Work out the finished part from the listing and answer in its coordinate system (mm). Face numbers are marked on the shaded views. A direction names the side the tool comes from. Round coordinates to 2 decimals unless told otherwise and drop trailing zeros. Write each loop counter-clockwise with the first axis right and the second up, starting at its lowest first coordinate (ties: lowest second). Pieces come first, ordered by that corner, then holes. Notation, with made-up numbers: (59, 39.5) -> (90, 39.5) arc R16 cw to (90, 52.5) -> close; hole circle Ø10 at (86.5, -39.75). An arc over 180 degrees is marked (long way). One line per item, written item: value.
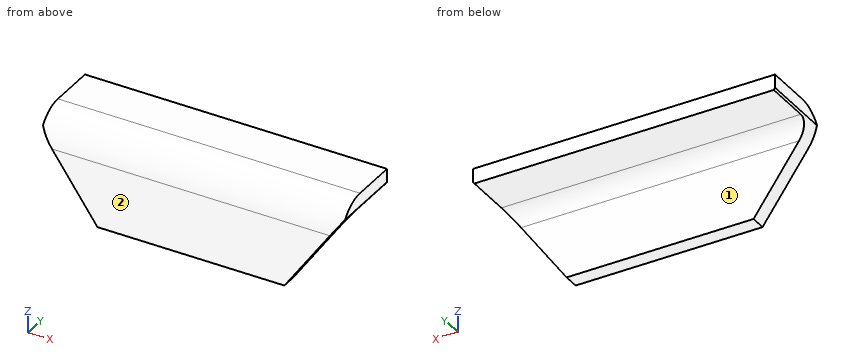
```python
from build123d import *

# Parameters (mm, degrees)
SKETCH1_W                    = 158
SKETCH1_H                    = 50
BASE_FLANGE1_DEPTH           = 8
EDGE_FLANGE1_STRIP_W         = 48
EDGE_FLANGE1_STRIP_H         = 8
EDGE_FLANGE1_STRIP_CUT_DEPTH = 158
EDGE_FLANGE1_DEPTH           = 158
CHAMFER1_SIZE                = 43
CHAMFER1_SIZE2               = 30.108924143
MIRROR2_START                = 54.388635645
MIRROR2_OUTLINE_W            = 56
MIRROR2_OUTLINE_H            = 41
MIRROR2_DEPTH                = 24.663786763


# Read off the part's stored shape, not the designer's step: Mirror2
# Sheet-metal steps are written as plain solids
with BuildPart() as part:
    # Sketch1 → Base-Flange1 (new body)
    with BuildSketch(Plane(origin=(0, 0, 0), x_dir=(1, 0, 0), z_dir=(0, 1, 0))):
        Rectangle(SKETCH1_W, SKETCH1_H)
    extrude(amount=-BASE_FLANGE1_DEPTH)

    # Edge-Flange1 strip (across the edge) → Edge-Flange1 strip cut (cut)
    with BuildSketch(Plane(origin=(-79, 0, 25), x_dir=(0, 0, -1), z_dir=(1, 0, 0))):
        with Locations((-8, -4)):
            Rectangle(EDGE_FLANGE1_STRIP_W, EDGE_FLANGE1_STRIP_H)
    extrude(amount=EDGE_FLANGE1_STRIP_CUT_DEPTH, mode=Mode.SUBTRACT)

    # Edge-Flange1 section (across the edge) → Edge-Flange1 (add)
    with BuildSketch(Plane(origin=(-79, 0, 25), x_dir=(0, 0, -1), z_dir=(1, 0, 0))):
        with BuildLine():
            Line((0, 8), (0, 32))
            Line((0, 32), (8, 32))
            Line((8, 32), (8, 8))
            ThreePointArc((8, 8), (10.343145751, 2.343145751), (16, 0))
            Line((16, 0), (16, -8))
            ThreePointArc((16, -8), (4.686291501, -3.313708499), (0, 8))
        make_face()
    extrude(amount=EDGE_FLANGE1_DEPTH)

    # Chamfer1
    chamfer1_edges = [part.edges().sort_by_distance(p)[0] for p in [
        (-79, -4, -25),
    ]]
    chamfer1_side = [part.faces().sort_by_distance(p)[0] for p in [
        (-79, -0.640312424, -8),
    ]]
    chamfer(chamfer1_edges, length=CHAMFER1_SIZE, length2=CHAMFER1_SIZE2, reference=chamfer1_side[0])

    # Mirror2 outline → Mirror2 (cut)
    with BuildSketch(Plane(origin=(0, 0, 0), x_dir=(0.5735764363510512, 0, 0.8191520442889882), z_dir=(0.8191520442889882, 0, -0.5735764363510512)).offset(MIRROR2_START)):
        with Locations((34, -12.5)):
            Rectangle(MIRROR2_OUTLINE_W, MIRROR2_OUTLINE_H)
    extrude(amount=MIRROR2_DEPTH, mode=Mode.SUBTRACT)


solid = part.part
```
(1) Find section C-C on y = 22.5. Give the vertices of the cut face in (x, z).
Reported:
outline: (-79, 18) -> (-78.3, 17) -> (78.3, 17) -> (79, 18) -> (79, 25) -> (-79, 25) -> close
(2) Find section D-D on z = -17.5. Give the vertices of the cut face in (x, y), plus the area to 3 significant figures.
Reported:
outline: (-54.14, -8) -> (54.14, -8) -> (54.14, 0) -> (-54.14, 0) -> close
area: 866 mm2
(3) Find section A-A on x = 18. Give the vertices of the cut face in (y, z), plus the area to 3 significant figures.
Reported:
outline: (-8, -25) -> (0, -25) -> (0, 9) arc R8 cw to (8, 17) -> (32, 17) -> (32, 25) -> (8, 25) arc R16 ccw to (-8, 9) -> close
area: 615 mm2
(4) Flat-ended cylindrical pins translate along their axes: pin 1 Ø10 at (y, z) = (-0.5, 8) entering from +X; pin 2 Ø8 at (x, z) = (-24.5, 6.5) entering from +Y; pin 3 Ø2 at (y, z) = (-3.5, 16) entering from +X. Find the tip coordinate at first contact, or state that the pin passes through.
Reported:
pin 1: stops at x = 75.5
pin 2: stops at y = 0.14
pin 3: stops at x = 78.3
(5) Find section B-B on y = -2. Give the vertices of the cut face in (x, z), plus the area to 3 significant figures.
Reported:
outline: (-79, 18) -> (-48.89, -25) -> (48.89, -25) -> (79, 18) -> (79, 21.49) -> (-79, 21.49) -> close
area: 6,050 mm2
(6) A tool of negligible diameter and unlimited length cuts with its end or side. For the marked faces 1 and 2, from which of +Z, -Z, +X, -X, +Y, -Y can it reach the whole face along a straight path? Write none if from no direction.
Reported:
face 1: -Z, +X, -X, +Y
face 2: +Z, -Z, +X, -X, -Y
(7) Consider probe 1 along Y at (x, z) = (-23, 18); probe 2 along Z at (x, y) = (-22.5, 13); probe 3 along Y at (x, z) = (15, -18). Determine where each line is inside the solid, lowest interval first.
Reported:
probe 1: y = -5.23 to 32
probe 2: z = 17 to 25
probe 3: y = -8 to 0
